Build history of the part. All positions in model axes, mm. Coordinates: 2 decimals unless noted, no trailing zeros. Write each loop counter-clockwise with the first axis right and the second up, starting at its lowest first coordinate (ties: lowest second). Pieces come first, ordered by that corner, then holes.
```python
from build123d import *

# Parameters (mm, degrees)
F0_W     = 44.45
F0_H     = 9.278706
F0_H_2   = 9.771294
F1_DEPTH = 25.4


with BuildPart() as f1:
    # F0 (on Front) → F1 (new body)
    with BuildSketch(Plane.XZ):
        with BuildLine():
            ThreePointArc((22.225, -19.173147), (41.275, -0.123147), (22.225, 18.926853))
            Line((22.225, 18.926853), (22.225, 9.648147))
            ThreePointArc((22.225, 9.648147), (28.960192, 6.858339), (31.75, 0.123147))
            ThreePointArc((31.75, 0.123147), (28.960192, -6.612045), (22.225, -9.401853))
            Line((22.225, -9.401853), (22.225, -19.173147))
        make_face()
        with Locations((0, 14.2875)):
            Rectangle(F0_W, F0_H)
        with Locations((0, -14.2875)):
            Rectangle(F0_W, F0_H_2)
        with BuildLine():
            Line((-22.225, 9.648147), (-22.225, 18.926853))
            ThreePointArc((-22.225, 18.926853), (-41.275, -0.123147), (-22.225, -19.173147))
            Line((-22.225, -19.173147), (-22.225, -9.401853))
            ThreePointArc((-22.225, -9.401853), (-31.75, 0.123147), (-22.225, 9.648147))
        make_face()
        with BuildLine():
            Line((22.225, 9.648147), (-22.225, 9.648147))
            ThreePointArc((-22.225, 9.648147), (-15.489808, 6.858339), (-12.7, 0.123147))
            ThreePointArc((-12.7, 0.123147), (-15.489808, -6.612045), (-22.225, -9.401853))
            Line((-22.225, -9.401853), (22.225, -9.401853))
            ThreePointArc((22.225, -9.401853), (12.7, 0.123147), (22.225, 9.648147))
        make_face()
    extrude(amount=F1_DEPTH)


solid = f1.part
```
1. Probe line 1 along X through (y, z) = (-11.25, -4); line 2 along Z through (x, y) = (-22, -14.75); line 3 along X through (y, z) = (-9.75, -7.5). List the from-to ranges inside material, lowest first.
Computed values:
line 1: x = -40.88 to -30.81, -13.64 to 13.64, 30.81 to 40.88
line 2: z = -19.17 to -9.4, 9.65 to 18.93
line 3: x = -39.79 to -27.94, -16.51 to 16.51, 27.94 to 39.79
2. Saw through at A-A on y = -7.5. List the corners of the cut face in (x, z) (3 decimals).
Computed values:
outline: (-22.225, -19.173) - (22.225, -19.173) arc R19.05 ccw to (22.225, 18.927) - (-22.225, 18.927) arc R19.05 ccw to start; hole circle Ø19.05 at (-22.225, 0.123); hole circle Ø19.05 at (22.225, 0.123)
3. Flat gauge pins, fed straight in: pin 1 (4 mm diameter, centred on y = -22, z = -9, fed in from -X); pin 2 (5 mm diameter, centred on y = -19, z = -1, fed in from +X) (3 decimals); pin 3 (3 mm diameter, centred on y = -9, z = 3.5, fed in from +X). Where does each tip first touch, or does it go through?
Computed values:
pin 1: stops at x = -39.99
pin 2: stops at x = 41.275
pin 3: stops at x = 41.16
4. Saw through at B-B on x = 28. List the corners of the cut face in (y, z), plus the area to 3 significant figures.
Computed values:
outline: (-25.4, -18.28) - (0, -18.28) - (0, -7.45) - (-25.4, -7.45) - close; (-25.4, 7.7) - (0, 7.7) - (0, 18.03) - (-25.4, 18.03) - close
area: 537 mm2
5. Mould opens along Y. For faces 1 (the face through (-1, -25.4, 0)), 2 (the face through (-41.27, -12.52, 0.3)), 3 (the face through (-1, 0, 0)) say: +Y half, -Y half, draft (parallel to the pull), parting line (faces both ways), or undercut.
Computed values:
face 1: -Y half
face 2: draft
face 3: +Y half
6. Saw through at C-C on z = 3. List the corners of the cut face in (x, y), plus the area to 3 significant figures.
Computed values:
outline: (-41.02, -25.4) - (-31.31, -25.4) - (-31.31, 0) - (-41.02, 0) - close; (-13.14, -25.4) - (13.14, -25.4) - (13.14, 0) - (-13.14, 0) - close; (31.31, -25.4) - (41.02, -25.4) - (41.02, 0) - (31.31, 0) - close
area: 1,160 mm2
7. Saw through at D-D on x = -25. List the corners of the cut face in (y, z).
Computed values:
outline: (-25.4, -18.97) - (0, -18.97) - (0, -8.99) - (-25.4, -8.99) - close; (-25.4, 9.23) - (0, 9.23) - (0, 18.72) - (-25.4, 18.72) - close
